Verification items for the finished model (mm, model axes). A direction names the side the tool comes from. Give positions to 0.01 mm unless a question says otherwise; leave off trailing zeros. Loops run counter-clockwise (first coordinate to the right, second up) from the corner with the lowest first, then second, coordinate; pieces in that order, holes last. Notation, with made-up numbers: (60, 1) -> (73, 1) arc R4 ccw to (73, 6) -> close; hole circle Ø1 at (58, -7). An arc over 180 degrees is marked (long way). Use one line per item in the form item = value. Start each with the question number.
from build123d import *

# Parameters (mm, degrees)
SKETCH1_W               = 285
SKETCH1_H               = 170
BOSS_EXTRUDE1_DEPTH     = 200
SHELL1_T                = -12
CUT_EXTRUDE1_DEPTH      = 359.399218749
CUT_EXTRUDE1_DEPTH_BACK = 359.399218749
SKETCH4_R               = 10
CUT_EXTRUDE2_DEPTH      = 12


with BuildPart() as part:
    # Sketch1 → Boss-Extrude1 (new body)
    with BuildSketch(Plane(origin=(0, 0, 0), x_dir=(1, 0, 0), z_dir=(0, 1, 0))):
        Rectangle(SKETCH1_W, SKETCH1_H)
    extrude(amount=BOSS_EXTRUDE1_DEPTH)

    # Shell1
    shell1_openings = [part.faces().sort_by_distance(p)[0] for p in [
        (0, 200, 0),
    ]]
    offset(amount=SHELL1_T, openings=shell1_openings, kind=Kind.INTERSECTION)

    # Sketch2 → Cut-Extrude1 (cut, two sides: drawn at the far end of the back side and taken through both)
    with BuildSketch(Plane(origin=(142.5, 0, 0), x_dir=(0, 0, -1), z_dir=(1, 0, 0)).offset(-CUT_EXTRUDE1_DEPTH_BACK)):
        with BuildLine():
            Line((-30, 190), (-30, 121))
            ThreePointArc((-30, 121), (0, 91), (30, 121))
            Line((30, 121), (30, 190))
            ThreePointArc((30, 190), (32.928932188, 197.071067812), (40, 200))
            Line((40, 200), (-40, 200))
            ThreePointArc((-40, 200), (-32.928932188, 197.071067812), (-30, 190))
        make_face()
    extrude(amount=CUT_EXTRUDE1_DEPTH + CUT_EXTRUDE1_DEPTH_BACK, mode=Mode.SUBTRACT)

    # Sketch4 → Cut-Extrude2 (cut)
    with BuildSketch(Plane.XY.offset(85)):
        with Locations((112.5, 105)):
            Circle(SKETCH4_R)
        with Locations((112.5, 75)):
            Circle(SKETCH4_R)
        with Locations((112.5, 45)):
            Circle(SKETCH4_R)
        with Locations((82.5, 95)):
            Circle(SKETCH4_R)
    extrude(amount=-CUT_EXTRUDE2_DEPTH, mode=Mode.SUBTRACT)


solid = part.part
Item 1: Tool access check on faces 1 (the cylindrical face through (110.33, 35.24, 79.08)), 2 (the cylindrical face through (136.42, 197.15, 33.01)), 3 (the flat face through (-1, 200, 74)), 4 (the flat face through (-2, 12, -1)). Record the directions out of +Z, -Z, +X, -X, +Y, -Y that give a thin tool (end or side, any length) a straight path to the whole face; none if there is none.
Item 2: Sectioned sample at A-A, the plane x = 112.5. Enter the section's corners in (y, z), and give its area (3 significant figures).
Item 3: Sectioned sample at B-B, the plane y = 126. Enter the section's corners in (x, z), and give its area (3 significant figures).
Item 4: Material ranges on line 1 (Y direction, x = 112.5, z = 78.25); line 2 (X direction, y = 171, z = -37); line 3 (Z direction, x = 44, y = 132), recorded low to high.
Item 5: Sectioned sample at D-D, the plane x = 7. Enter the section's corners in (y, z), and give its area (3 significant figures).
Item 6: Gauge pin test, flat ends, axial feed: pin 1 Ø1 at (x, z) = (64.5, -3) entering from +Y; pin 2 Ø16 at (x, y) = (112.5, 75) entering from +Z. Record the tip position at first contact, or that the pin passes through.
Item 7: Draft check along X on faces 5 (the flat face through (-2, 0, -1)), 6 (the flat face through (142.5, 76, 1)), 7 (the cylindrical face through (111.198, 114.915, 79.084)). Enter one of: +X half, -X half, draft (parallel to the pull), parting line (faces both ways), or undercut.
Item 8: Sectioned sample at C-C, the plane z = 0. Enter the section's corners in (x, y).
Outcome:
q1.face_1 = +Z
q1.face_2 = +X, -X, +Y
q1.face_3 = +Z, -Z, +X, -X, +Y
q1.face_4 = +Y
q2.outline = (0, -85) -> (200, -85) -> (200, -73) -> (12, -73) -> (12, 73) -> (35, 73) -> (35, 85) -> (0, 85) -> close; (55, 73) -> (65, 73) -> (65, 85) -> (55, 85) -> close; (85, 73) -> (95, 73) -> (95, 85) -> (85, 85) -> close; (115, 73) -> (200, 73) -> (200, 85) -> (115, 85) -> close
q2.area = 5,830 mm^2
q3.outline = (-142.5, -85) -> (142.5, -85) -> (142.5, -30) -> (130.5, -30) -> (130.5, -73) -> (-130.5, -73) -> (-130.5, -30) -> (-142.5, -30) -> close; (-142.5, 30) -> (-130.5, 30) -> (-130.5, 73) -> (130.5, 73) -> (130.5, 30) -> (142.5, 30) -> (142.5, 85) -> (-142.5, 85) -> close
q3.area = 8,900 mm^2
q4.line_1 = 0 to 35, 55 to 65, 85 to 95, 115 to 200
q4.line_2 = -142.5 to -130.5, 130.5 to 142.5
q4.line_3 = -85 to -73, 73 to 85
q5.outline = (0, -85) -> (200, -85) -> (200, -73) -> (12, -73) -> (12, 73) -> (200, 73) -> (200, 85) -> (0, 85) -> close
q5.area = 6,550 mm^2
q6.pin_1 = 12
q6.pin_2 = -73
q7.face_5 = draft
q7.face_6 = +X half
q7.face_7 = undercut
q8.outline = (-142.5, 0) -> (142.5, 0) -> (142.5, 91) -> (130.5, 91) -> (130.5, 12) -> (-130.5, 12) -> (-130.5, 91) -> (-142.5, 91) -> close
